Geometry: final body of the model. Coordinates: model frame, mm. Face numbers are marked on the shaded views. A direction names the side the tool comes from. Coordinates: 2 decimals unless noted, no trailing zeros. Write each loop counter-clockwise with the first axis right and the second up, starting at its lowest first coordinate (ties: lowest second). Pieces come first, ordered by that corner, then holes. Notation, with made-up numbers: (21, 73.5) -> (55, 73.5) arc R13 ccw to (55, 96.5) -> close; hole circle Ø7 at (33, -23). An arc over 180 degrees is marked (long way). One line per item, written item: value.
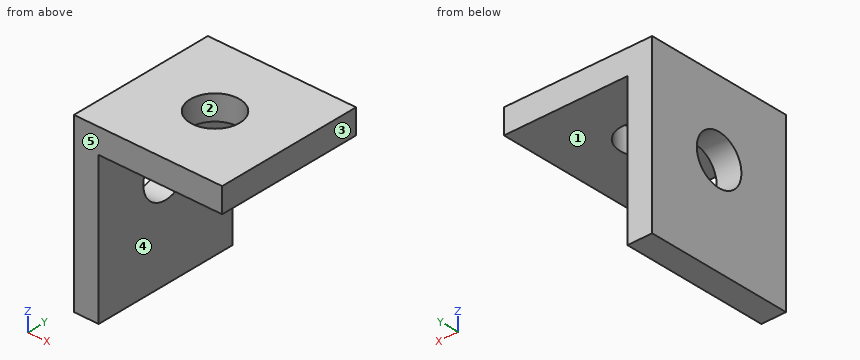
```python
from build123d import *

# Parameters (mm, degrees)
CROQUIS1_W              = 5
CROQUIS1_H              = 30
CROQUIS1_W_2            = 30
CROQUIS1_H_2            = 5
SALIENTE_EXTRUIR1_DEPTH = 30
CROQUIS2_R              = 5
CORTAR_EXTRUIR1_DEPTH   = 5
CROQUIS3_R              = 5
CORTAR_EXTRUIR2_DEPTH   = 5


with BuildPart() as part:
    # Croquis1 → Saliente-Extruir1 (new body)
    with BuildSketch(Plane(origin=(0, 0, 0), x_dir=(1, 0, 0), z_dir=(0, 1, 0))):
        with Locations((-12.5, 17.5)):
            Rectangle(CROQUIS1_W, CROQUIS1_H)
        Rectangle(CROQUIS1_W_2, CROQUIS1_H_2)
    extrude(amount=SALIENTE_EXTRUIR1_DEPTH)

    # Croquis2 → Cortar-Extruir1 (cut)
    with BuildSketch(Plane.XY.offset(2.5)):
        with Locations((0, 15)):
            Circle(CROQUIS2_R)
    extrude(amount=-CORTAR_EXTRUIR1_DEPTH, mode=Mode.SUBTRACT)

    # Croquis3 → Cortar-Extruir2 (cut)
    with BuildSketch(Plane.ZY.offset(15)):
        with Locations((-12.5, 15)):
            Circle(CROQUIS3_R)
    extrude(amount=-CORTAR_EXTRUIR2_DEPTH, mode=Mode.SUBTRACT)


solid = part.part
```
(1) Section D-D (z = 0.5). Return the cut outline in (x, y), then the cut area to 3 significant figures.
Responses:
outline: (-15, 0) -> (15, 0) -> (15, 30) -> (-15, 30) -> close; hole circle Ø10 at (0, 15)
area: 821 mm2
(2) Section B-B (z = -12.5). Return the cut outline in (x, y).
Responses:
outline: (-15, 0) -> (-10, 0) -> (-10, 10) -> (-15, 10) -> close; (-15, 20) -> (-10, 20) -> (-10, 30) -> (-15, 30) -> close
(3) Line query: line 1 (Y direction, x = -13.5, z = -12.5); line 2 (X direction, y = 6.75, z = -5); line 3 (Z direction, x = -2.5, y = 27.5). Output: solid intervals per line, ascending. Write a range as [from, to].
Responses:
line 1: y = [0, 10], [20, 30]
line 2: x = [-15, -10]
line 3: z = [-2.5, 2.5]
(4) First-contact query: pin 1 (8 mm diameter, centred on x = 0, y = 15, fed in from +Z); pin 2 (10 mm diameter, centred on y = 25.5, z = -20, fed in from +X); pin 3 (1.5 mm diameter, centred on x = 6, y = 16.5, fed in from -Z). Flat tips, straight axial feed; report the tip coordinate or a pass-through.
Responses:
pin 1: passes through
pin 2: stops at x = -10
pin 3: stops at z = -2.5
(5) Pull-direction query (X, two-part tool) for the marked faces 1, 2 and 3; classes: released by +X, released by -X, zero draft, split by the parting line, or undercut.
Responses:
face 1: zero draft
face 2: undercut
face 3: released by +X
(6) Reachability of the marked faces 4 and 5 from +Z, -Z, +X, -X, +Y, -Y: full face, straight path, thin tool, end or side. Return the list, or none.
Responses:
face 4: -Z, +X, +Y, -Y
face 5: +Z, -Z, +X, -X, -Y
(7) Section A-A (y = 15). Return the cut outline in (x, z).
Responses:
outline: (-15, -32.5) -> (-10, -32.5) -> (-10, -17.5) -> (-15, -17.5) -> close; (-15, -7.5) -> (-10, -7.5) -> (-10, -2.5) -> (-5, -2.5) -> (-5, 2.5) -> (-15, 2.5) -> close; (5, -2.5) -> (15, -2.5) -> (15, 2.5) -> (5, 2.5) -> close
(8) Section C-C (x = 0). Return the cut outline in (y, z).
Responses:
outline: (0, -2.5) -> (10, -2.5) -> (10, 2.5) -> (0, 2.5) -> close; (20, -2.5) -> (30, -2.5) -> (30, 2.5) -> (20, 2.5) -> close
